from build123d import *

# Parameters (mm, degrees)
DODANIE_WYCI_GNI_CIE1_DEPTH      = 5
DODANIE_WYCI_GNI_CIE1_DEPTH_BACK = 5
SZKIC1_R                         = 7.5
SZKIC1_R_2                       = 14
SZKIC1_R_3                       = 17.5
SZKIC1_R_4                       = 5
ZAOKR_GLENIE1_R                  = 3
ZAOKR_GLENIE2_R                  = 3


with BuildPart() as part:
    # Szkic1 → Dodanie-wyci_gni_cie1 (new, two sides: drawn at the far end of the back side and taken through both)
    with BuildSketch(Plane(origin=(0, 0, 0), x_dir=(0, 0, -1), z_dir=(1, 0, 0)).offset(-DODANIE_WYCI_GNI_CIE1_DEPTH_BACK)):
        with BuildLine():
            Line((-25, 0), (-25, 68.867513459))
            Line((-25, 68.867513459), (44.841238994, 152.101060942))
            Line((44.841238994, 152.101060942), (62.16174707, 142.101060942))
            Line((62.16174707, 142.101060942), (25, 40))
            Line((25, 40), (25, 0))
            ThreePointArc((25, 0), (0, -25), (-25, 0))
        make_face()
        with Locations((39.751493032, 123.285362338)):
            Circle(SZKIC1_R, mode=Mode.SUBTRACT)
        with Locations((24.751493032, 97.304600224)):
            Circle(SZKIC1_R_2, mode=Mode.SUBTRACT)
        with Locations((4.751493032, 62.663584073)):
            Circle(SZKIC1_R_3, mode=Mode.SUBTRACT)
        with Locations((0, -7)):
            Circle(SZKIC1_R_4, mode=Mode.SUBTRACT)
    extrude(amount=DODANIE_WYCI_GNI_CIE1_DEPTH + DODANIE_WYCI_GNI_CIE1_DEPTH_BACK)

    # Szkic3 → Obr_t1 (revolve)
    with BuildSketch(Plane(origin=(0, 0, 0), x_dir=(0, 0, -1), z_dir=(1, 0, 0)), mode=Mode.PRIVATE) as obr_t1_sk:
        Polygon((40.511111975, 154.601060942), (53.501493032, 147.101060942), (111.501493032, 247.560007781), (98.511111975, 255.060007781), (94.511111975, 248.131804551), (90.180984956, 250.631804551), (40.180984956, 164.029264172), (44.511111975, 161.529264172), align=None)
    revolve(obr_t1_sk.sketch.rotate(Axis((0, 147.101060942, -53.501493032), (0, 0.8660254037844385, -0.5000000000000003)), 180), axis=Axis((0, 147.101060942, -53.501493032), (0, 0.8660254037844385, -0.5000000000000003)))

    # Zaokr_glenie1
    zaokr_glenie1_edges = [part.edges().sort_by_distance(p)[0] for p in [
        (0, 154.601060942, -40.511111975),
        (0, 255.060007781, -98.511111975),
    ]]
    fillet(zaokr_glenie1_edges, radius=ZAOKR_GLENIE1_R)

    # Zaokr_glenie2
    zaokr_glenie2_edges = [part.edges().sort_by_distance(p)[0] for p in [
        (0, 250.631804551, -90.180984956),
        (0, 164.029264172, -40.180984956),
    ]]
    fillet(zaokr_glenie2_edges, radius=ZAOKR_GLENIE2_R)


solid = part.part
The listing builds one solid part. Answer for the finished solid, in the listing's coordinates (mm). A direction names the side the tool comes from. Round coordinates to 2 decimals unless told otherwise and drop trailing zeros. Write each loop counter-clockwise with the first axis right and the second up, starting at its lowest first coordinate (ties: lowest second). Pieces come first, ordered by that corner, then holes. Notation, with made-up numbers: (49.5, -32) - (80.5, -32) arc R15 ccw to (80.5, -8) - close; hole circle Ø7 at (20, 78). An arc over 180 degrees is marked (long way). Use a Markdown table: item, result. Add a question column.
1. Consider line 1 (Y direction, x = 2, z = 0); line 2 (X direction, y = 47.5, z = 16.5); line 3 (Y direction, x = 3, z = 7). Determine where each line is inside the solid, lowest interval first.
2. Flat-ended cylindrical pins translate along their axes: P1, Ø1.5, axis at x = -4, y = 136.5, coming from the -Z side; P2, Ø3, axis at x = 0, y = 11.5, coming from the -Z side; P3, Ø5, axis at x = 9.5, y = 155.5, coming from the -Z side. Find the tip coordinate at first contact, or state that the pin passes through.
3. The part is cut by section C-C (y = 104). Write down the section's boundary in (x, z).
4. For a pull along Y with two mould halves and no side action, classify faces 1 (the face through (-0.07, 91.765, -43.841)), 2 (the face through (0, -3, -3)), 3 (the face through (5, 45, -10)) as +Y half, -Y half, draft (parallel to the pull), parting line (faces both ways), or undercut.
5. The part is cut by section B-B (z = 0). Write down the section's boundary in (x, y).
6. The part is cut by section A-A (y = -7). Write down the section's boundary in (x, z), and give its area (3 significant figures).
7. A tool of negligible diameter and unlimited length cuts with its end or side. For faces 4 (the face through (12.51, 149.66, -65.07)), 5 (the face through (-0.168, 247.476, -111.647)), 6 (the face through (0, 20, -25)), from which of +Z, -Z, +X, -X, +Y, -Y can it reach the whole face along a straight path? Write none if from no direction.
Reported:
| question | item | result |
|---|---|---|
| 1 | line 1 | -25 to -12, -2 to 45.82, 79.51 to 98.66 |
| 1 | line 2 | -5 to 5 |
| 1 | line 3 | -24 to 49.7, 75.63 to 90.32 |
| 2 | P1 | z = -60.4 |
| 2 | P2 | z = -25 |
| 2 | P3 | z = -80.68 |
| 3 | outline | (-5, -48.29) - (5, -48.29) - (5, -37.05) - (-5, -37.05) - close; (-5, -12.46) - (5, -12.46) - (5, -4.48) - (-5, -4.48) - close |
| 4 | face 1 | -Y half |
| 4 | face 2 | undercut |
| 4 | face 3 | draft |
| 5 | outline | (-5, -25) - (5, -25) - (5, -12) - (-5, -12) - close; (-5, -2) - (5, -2) - (5, 45.82) - (-5, 45.82) - close; (-5, 79.51) - (5, 79.51) - (5, 98.66) - (-5, 98.66) - close |
| 6 | outline | (-5, -24) - (5, -24) - (5, -5) - (-5, -5) - close; (-5, 5) - (5, 5) - (5, 24) - (-5, 24) - close |
| 6 | area | 380 mm^2 |
| 7 | face 4 | none |
| 7 | face 5 | -Z, +X, -X, +Y |
| 7 | face 6 | -Z, +X, -X, -Y |
